```python
from build123d import *
from build123d import SkipClean  # not in build123d's __all__

# Parameters (mm, degrees)
F0_R     = 260
F1_DEPTH = 10
F2_DEPTH = 900
F3_DEPTH = 500
F4_DEPTH = 450
F5_R     = 24.5282559267
F6_DEPTH = 100
F8_DEPTH = 100


# Not quite as in the source:
# - after a boolean that leaves OpenCascade's solid faulty, fix() repairs it


with BuildPart() as f1:
    # F0 (on Top) → F1 (new body)
    with BuildSketch(Plane.XY):
        with BuildLine():
            ThreePointArc((263.8181191655, -25), (264.7043648855, -12.5139606271), (265, 0))
            ThreePointArc((265, 0), (264.7043648855, 12.5139606271), (263.8181191655, 25))
            ThreePointArc((263.8181191655, 25), (0, 265), (-263.8181191655, 25))
            ThreePointArc((-263.8181191655, 25), (-264.7043648855, 12.5139606271), (-265, 0))
            ThreePointArc((-265, 0), (-264.7043648855, -12.5139606271), (-263.8181191655, -25))
            ThreePointArc((-263.8181191655, -25), (0, -265), (263.8181191655, -25))
        make_face()
        Circle(F0_R, mode=Mode.SUBTRACT)
        Circle(F0_R)
    extrude(amount=F1_DEPTH)

    # F0 (on Top) → F2 (join)
    with BuildSketch(Plane.XY):
        with BuildLine():
            ThreePointArc((263.8181191655, -25), (264.7043648855, -12.5139606271), (265, 0))
            ThreePointArc((265, 0), (264.7043648855, 12.5139606271), (263.8181191655, 25))
            ThreePointArc((263.8181191655, 25), (0, 265), (-263.8181191655, 25))
            ThreePointArc((-263.8181191655, 25), (-264.7043648855, 12.5139606271), (-265, 0))
            ThreePointArc((-265, 0), (-264.7043648855, -12.5139606271), (-263.8181191655, -25))
            ThreePointArc((-263.8181191655, -25), (0, -265), (263.8181191655, -25))
        make_face()
        Circle(F0_R, mode=Mode.SUBTRACT)
    extrude(amount=F2_DEPTH)

    # F0 (on Top) → F3 (join)
    with BuildSketch(Plane.XY):
        with BuildLine():
            Line((275, 0), (265, 0))
            ThreePointArc((265, 0), (264.7043648855, -12.5139606271), (263.8181191655, -25))
            Line((263.8181191655, -25), (275, -25))
            Line((275, -25), (275, 0))
        make_face()
        with BuildLine():
            ThreePointArc((263.8181191655, 25), (264.7043648855, 12.5139606271), (265, 0))
            Line((265, 0), (275, 0))
            Line((275, 0), (275, 25))
            Line((275, 25), (263.8181191655, 25))
        make_face()
        with BuildLine():
            ThreePointArc((-265, 0), (-264.7043648855, 12.5139606271), (-263.8181191655, 25))
            Line((-263.8181191655, 25), (-275, 25))
            Line((-275, 25), (-275, 0))
            Line((-275, 0), (-265, 0))
        make_face()
        with BuildLine():
            Line((-275, -25), (-263.8181191655, -25))
            ThreePointArc((-263.8181191655, -25), (-264.7043648855, -12.5139606271), (-265, 0))
            Line((-265, 0), (-275, 0))
            Line((-275, 0), (-275, -25))
        make_face()
    extrude(amount=F3_DEPTH)

    # F0 (on Top) → F4 (cut)
    with BuildSketch(Plane.XY):
        with BuildLine():
            ThreePointArc((263.8181191655, 25), (264.7043648855, 12.5139606271), (265, 0))
            Line((265, 0), (275, 0))
            Line((275, 0), (275, 25))
            Line((275, 25), (263.8181191655, 25))
        make_face()
        with BuildLine():
            Line((275, 0), (265, 0))
            ThreePointArc((265, 0), (264.7043648855, -12.5139606271), (263.8181191655, -25))
            Line((263.8181191655, -25), (275, -25))
            Line((275, -25), (275, 0))
        make_face()
        with BuildLine():
            ThreePointArc((-265, 0), (-264.7043648855, 12.5139606271), (-263.8181191655, 25))
            Line((-263.8181191655, 25), (-275, 25))
            Line((-275, 25), (-275, 0))
            Line((-275, 0), (-265, 0))
        make_face()
        with BuildLine():
            Line((-275, -25), (-263.8181191655, -25))
            ThreePointArc((-263.8181191655, -25), (-264.7043648855, -12.5139606271), (-265, 0))
            Line((-265, 0), (-275, 0))
            Line((-275, 0), (-275, -25))
        make_face()
    with SkipClean():  # cleaning this boolean's faces spoils the solid; the shape is the same uncleaned
        extrude(amount=F4_DEPTH, mode=Mode.SUBTRACT)

    # F5 (on face) → F6 (join)
    with BuildSketch(Plane(origin=(-275, 0, 0), x_dir=(0, -1, 0), z_dir=(-1, 0, 0))):
        with Locations((0, 475)):
            Circle(F5_R)
    extrude(amount=F6_DEPTH)

    add(f1.part.fix(), mode=Mode.REPLACE)

    # F7 (on face) → F8 (join)
    with BuildSketch(Plane.YZ.offset(275)):
        with BuildLine():
            Line((17.6776695297, 492.6776695297), (0, 475))
            Line((0, 475), (17.6776695297, 457.3223304703))
            ThreePointArc((17.6776695297, 457.3223304703), (23.0969883128, 465.4329141909), (25, 475))
            ThreePointArc((25, 475), (23.0969883128, 484.5670858091), (17.6776695297, 492.6776695297))
        make_face()
        with BuildLine():
            ThreePointArc((2.731e-07, 500), (-9.567085683, 498.096988365), (-17.6776695297, 492.6776695297))
            Line((-17.6776695297, 492.6776695297), (0, 475))
            Line((0, 475), (17.6776695297, 492.6776695297))
            ThreePointArc((17.6776695297, 492.6776695297), (9.5670859353, 498.0969882605), (2.731e-07, 500))
        make_face()
        with BuildLine():
            Line((0, 475), (-17.6776695297, 492.6776695297))
            ThreePointArc((-17.6776695297, 492.6776695297), (-23.0969883128, 484.5670858091), (-25, 475))
            ThreePointArc((-25, 475), (-23.0969883128, 465.4329141909), (-17.6776695297, 457.3223304703))
            Line((-17.6776695297, 457.3223304703), (0, 475))
        make_face()
        with BuildLine():
            Line((17.6776695297, 457.3223304703), (0, 475))
            Line((0, 475), (-17.6776695297, 457.3223304703))
            ThreePointArc((-17.6776695297, 457.3223304703), (-9.5670857461, 451.9030116611), (1.365e-07, 450))
            ThreePointArc((1.365e-07, 450), (9.5670858722, 451.9030117133), (17.6776695297, 457.3223304703))
        make_face()
    extrude(amount=F8_DEPTH)


solid = f1.part
```
The listing builds one solid part. Answer for the finished solid, in the listing's coordinates (mm). A direction names the side the tool comes from. Round coordinates to 2 decimals unless told otherwise and drop trailing zeros. Loops run counter-clockwise (first coordinate to the right, second up) from the corner with the lowest first, then second, coordinate; pieces in that order, holes last.
Q1. Section A-A, the plane z = 233 is taken. Determine the outline of the cut face in (x, y).
Q2. Find the intervals of material crossed by line 1 (Y direction, x = 0, z = 615); line 2 (X direction, y = 0, z = 466), in increasing order.
Q3. Given pin 1 Ø3.5 at (x, z) = (266.5, 480.5) entering from +Y; pin 2 Ø10 at (y, z) = (96.5, 408) entering from -X; pin 3 Ø6 at (x, z) = (-67.5, 385.5) entering from +Y, each flat-ended and moving along its own axis, determine where each tip first touches the part or whether it passes through.
Q4. Which of the six approach directions +Z, -Z, +X, -X, +Y, -Y give full straight-line access (tool end or side, diameter ignored) to faces 1 (the face through (247.994, 78.097, 448.77)), 2 (the face through (275, 19, 455)), 3 (the face through (-324.3, 5.317, 451.055))?
Q5. Section C-C, the plane y = -197 is taken. Determine the outline of the cut face in (x, z), then the cut area to 3 significant figures.
Q6. For a pull along X with two mould halves and no side action, classify faces 4 (the face through (195, -175, 900)), 5 (the face through (-4, 4, 10)), 6 (the face through (375, 0, 475)) as released by +X, released by -X, zero draft, split by the parting line, or undercut.
Q7. Section B-B, the plane x = 0 is taken. Determine the outline of the cut face in (y, z), then the cut area to 3 significant figures.
Completed:
1. outline: circle Ø530 at (0, 0); hole circle Ø520 at (0, 0)
2. line 1: y = -265 to -260, 260 to 265
2. line 2: x = -375 to -260, 260 to 375
3. pin 1: stops at y = 25
3. pin 2: stops at x = -248.7
3. pin 3: stops at y = 257.03
4. face 1: +Z
4. face 2: -Z, +X, +Y
4. face 3: -X
5. outline: (-177.25, 0) - (177.25, 0) - (177.25, 900) - (169.68, 900) - (169.68, 10) - (-169.68, 10) - (-169.68, 900) - (-177.25, 900) - close
5. area: 17,000 mm2
6. face 4: zero draft
6. face 5: undercut
6. face 6: released by +X
7. outline: (-265, 0) - (265, 0) - (265, 900) - (260, 900) - (260, 10) - (-260, 10) - (-260, 900) - (-265, 900) - close
7. area: 14,200 mm2
